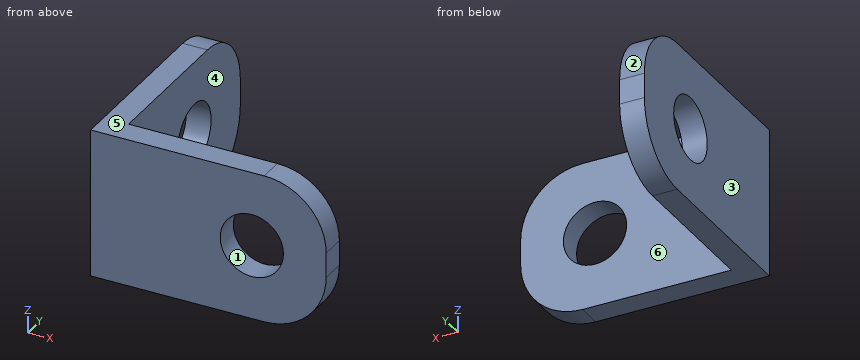
from build123d import *

# Parameters (mm, degrees)
EXTRUDE_1_DEPTH     = 12
SKETCH_2_R          = 2.55
CUT_EXTRUDE_1_DEPTH = 3
SKETCH_3_R          = 2.55
CUT_EXTRUDE_2_DEPTH = 3


with BuildPart() as part:
    # Эскиз1 → Бобышка-Вытянуть1 (new body)
    with BuildSketch(Plane.XY):
        Polygon((0, 0), (0, 19), (2, 19), (2, 2), (19, 2), (19, 0), align=None)
    extrude(amount=EXTRUDE_1_DEPTH)

    # Эскиз2 → Вырез-Вытянуть1 (cut, through all)
    with BuildSketch(Plane(origin=(2, 0, 0), x_dir=(0, 0, -1), z_dir=(1, 0, 0))):
        with Locations((-6, 12)):
            Circle(SKETCH_2_R)
        with BuildLine():
            Line((-12, 14), (-12, 19))
            Line((-12, 19), (-7, 19))
            ThreePointArc((-7, 19), (-10.535533906, 17.535533906), (-12, 14))
        make_face()
        with BuildLine():
            Line((0, 14), (0, 19))
            Line((0, 19), (-5, 19))
            ThreePointArc((-5, 19), (-1.464466094, 17.535533906), (0, 14))
        make_face()
    extrude(amount=-CUT_EXTRUDE_1_DEPTH, mode=Mode.SUBTRACT)

    # Эскиз3 → Вырез-Вытянуть2 (cut, through all)
    with BuildSketch(Plane(origin=(0, 2, 0), x_dir=(1, 0, 0), z_dir=(0, 1, 0))):
        with Locations((13, -6)):
            Circle(SKETCH_3_R)
        with BuildLine():
            Line((14, 0), (19, 0))
            Line((19, 0), (19, -5))
            ThreePointArc((19, -5), (17.535533906, -1.464466094), (14, 0))
        make_face()
        with BuildLine():
            Line((14, -12), (19, -12))
            Line((19, -12), (19, -7))
            ThreePointArc((19, -7), (17.535533906, -10.535533906), (14, -12))
        make_face()
    extrude(amount=-CUT_EXTRUDE_2_DEPTH, mode=Mode.SUBTRACT)


solid = part.part
Check sheet for the modelled part. Datum: model origin and axes. Units: mm. Face numbers are marked on the shaded views. A direction names the side the tool comes from. Round coordinates to 2 decimals unless told otherwise and drop trailing zeros. Order: outer loops, then holes, each group sorted by start corner. A loop starts at its lowest first (then second) coordinate and runs counter-clockwise, first axis right, second up.
(1) Cross-section at D-D, the plane z = 2. Enter the section's corners in (x, y), and give its area (3 significant figures).
(2) Access from +Z, -Z, +X, -X, +Y, -Y to the whole of each face (thin tool, end or side, straight path). Record for the marked faces 5 and 6.
(3) Go/stop test with flat-tipped pins: P1, Ø6.5, axis at y = 12, z = 6, coming from the -X side; P2, Ø1, axis at x = 13, z = 9, coming from the +Y side. Record where each tip stops, or that it passes through.
(4) Draft check along X on the marked faces 1, 2, 3 and 4. Enter one of: pulls with the +X half, pulls with the -X half, needs draft (parallel to the pull), parting line crosses it, or undercut.
(5) Scan lines: probe 1 along X at (y, z) = (1.5, 6); probe 2 along Y at (x, z) = (1.4, 6); probe 3 along Z at (x, y) = (13, 0.7). Record each from-to range of solid material in increasing order.
(6) Cross-section at A-A, the plane y = 12. Enter the section's corners in (x, z), and give its area (3 significant figures).
(7) Cross-section at C-C, the plane z = 6. Enter the section's corners in (x, y), and give its area (3 significant figures).
Check sheet entries:
1. outline: (0, 0) - (18, 0) - (18, 2) - (2, 2) - (2, 18) - (0, 18) - close
1. area: 68.0 mm2
2. face 5: +Z, +X, -X, +Y, -Y
2. face 6: +Z, -Z, +X, +Y
3. P1: stops at x = 0
3. P2: stops at y = 2
4. face 1: undercut
4. face 2: needs draft
4. face 3: pulls with the -X half
4. face 4: pulls with the +X half
5. probe 1: x = 0 to 10.45, 15.55 to 19
5. probe 2: y = 0 to 9.45, 14.55 to 19
5. probe 3: z = 0 to 3.45, 8.55 to 12
6. outline: (0, 0) - (2, 0) - (2, 3.45) - (0, 3.45) - close; (0, 8.55) - (2, 8.55) - (2, 12) - (0, 12) - close
6. area: 13.8 mm2
7. outline: (0, 0) - (10.45, 0) - (10.45, 2) - (2, 2) - (2, 9.45) - (0, 9.45) - close; (0, 14.55) - (2, 14.55) - (2, 19) - (0, 19) - close; (15.55, 0) - (19, 0) - (19, 2) - (15.55, 2) - close
7. area: 51.6 mm2
